from build123d import *

# Parameters (mm, degrees)
F1_DEPTH = 3.175
F2_R     = 5.08
F3_R     = 0.508


with BuildPart() as f1:
    # F0 (on Top) → F1 (new body)
    with BuildSketch(Plane.XY):
        with BuildLine():
            Line((-30.841844, 43.311745), (-30.841844, -61.686775))
            Line((-30.841844, -61.686775), (-18.141844, -61.686775))
            Line((-18.141844, -61.686775), (-5.441844, -23.358175))
            Line((-5.441844, -23.358175), (-5.441844, -10.658175))
            Line((-5.441844, -10.658175), (-18.141844, -10.658175))
            ThreePointArc((-18.141844, -10.658175), (-22.109324, -6.690695), (-18.141844, -2.723215))
            Line((-18.141844, -2.723215), (-5.441844, -2.723215))
            Line((-5.441844, -2.723215), (-5.441844, 0.451785))
            Line((-5.441844, 0.451785), (-18.141844, 0.451785))
            ThreePointArc((-18.141844, 0.451785), (-23.696824, 6.006765), (-18.141844, 11.561745))
            Line((-18.141844, 11.561745), (-5.441844, 11.561745))
            Line((-5.441844, 11.561745), (-5.441844, 17.911745))
            Line((-5.441844, 17.911745), (-18.141844, 17.911745))
            ThreePointArc((-18.141844, 17.911745), (-21.316844, 21.086745), (-18.141844, 24.261745))
            Line((-18.141844, 24.261745), (-5.441844, 24.261745))
            Line((-5.441844, 24.261745), (-5.441844, 27.436745))
            Line((-5.441844, 27.436745), (-18.141844, 27.436745))
            ThreePointArc((-18.141844, 27.436745), (-22.904344, 32.199245), (-18.141844, 36.961745))
            Line((-18.141844, 36.961745), (-5.441844, 36.961745))
            Line((-5.441844, 36.961745), (-5.441844, 43.311745))
            Line((-5.441844, 43.311745), (-30.841844, 43.311745))
        make_face()
    extrude(amount=F1_DEPTH)

    # F2
    f2_edges = [f1.edges().sort_by_distance(p)[0] for p in [
        (-18.141844, -61.686775, 1.5875),
        (-5.441844, -23.358175, 1.5875),
        (-30.841844, -61.686775, 1.5875),
        (-5.441844, 43.311745, 1.5875),
        (-30.841844, 43.311745, 1.5875),
    ]]
    fillet(f2_edges, radius=F2_R)

    # F3
    f3_edges = [f1.edges().sort_by_distance(p)[0] for p in [
        (-5.441844, -10.658175, 1.5875),
        (-5.441844, -2.723215, 1.5875),
        (-5.441844, 0.451785, 1.5875),
        (-5.441844, 11.561745, 1.5875),
        (-5.441844, 17.911745, 1.5875),
        (-5.441844, 24.261745, 1.5875),
        (-5.441844, 27.436745, 1.5875),
        (-5.441844, 36.961745, 1.5875),
    ]]
    fillet(f3_edges, radius=F3_R)


solid = f1.part
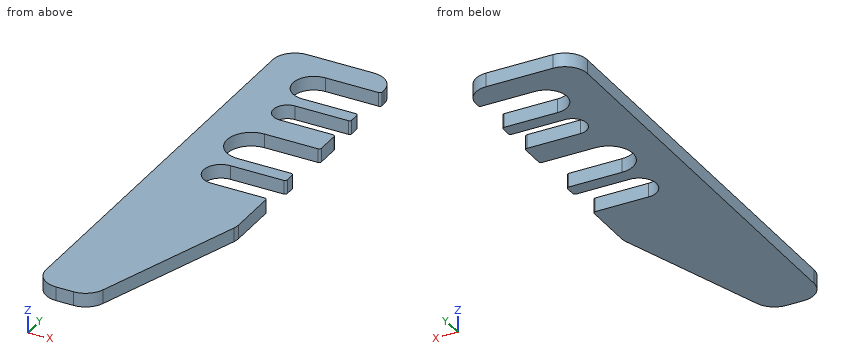
Read the model definition and answer for the solid it produces. Units are mm, in the model's axes. Coordinates: 2 decimals unless noted, no trailing zeros. Write each loop counter-clockwise with the first axis right and the second up, starting at its lowest first coordinate (ties: lowest second). Pieces come first, ordered by that corner, then holes. Notation, with made-up numbers: (-3, 45.25) -> (29, 45.25) arc R22 cw to (29, 82.25) -> close; hole circle Ø7 at (-28.5, -10). An arc over 180 degrees is marked (long way). Return JSON: item names as keys, results as strings.
(1) Consider line 1 along Y through (x, z) = (-19.75, 2.3); line 2 along Y through (x, z) = (-17.5, 2); line 3 along Y through (x, z) = (-21.75, 1.7). Determine where each line is inside the solid, lowest interval first. Write a range as from..to.
Answers below:
{"line 1": "-61.25..-10.32, -3.06..0.69, 11.32..18.35, 23.82..27.72, 36.68..43.31", "line 2": "-59.3..-10.66, -2.72..0.45, 11.56..17.91, 24.26..27.44, 36.96..43.31", "line 3": "-61.69..-8.34, -5.04..1.78, 10.23..29.09, 35.31..43.31"}
(2) Each of these flat-tipped pins is pushed along its axis until it touches: P1, Ø6, axis at x = -10.5, y = 11, coming from the +Z side (3 decimals); P2, Ø1, axis at x = -21, z = 2, coming from the -Y side. Where does it stop, or does it pass through?
Answers below:
{"P1": "z = 3.175", "P2": "y = -61.68"}
(3) The part is cut by section A-A on x = -20.25. Give the vertices of the cut face in (y, z) (3 decimals), then the cut area to 3 significant figures.
Answers below:
{"outline": "(-61.441, 0) -> (-10.052, 0) -> (-10.052, 3.175) -> (-61.441, 3.175) -> close; (-3.33, 0) -> (0.867, 0) -> (0.867, 3.175) -> (-3.33, 3.175) -> close; (11.146, 0) -> (18.713, 0) -> (18.713, 3.175) -> (11.146, 3.175) -> close; (23.461, 0) -> (27.929, 0) -> (27.929, 3.175) -> (23.461, 3.175) -> close; (36.47, 0) -> (43.312, 0) -> (43.312, 3.175) -> (36.47, 3.175) -> close", "area": "236 mm^2"}
(4) The part is cut by section C-C on x = -8.75. Give the vertices of the cut face in (y, z) (3 decimals), then the cut area to 3 significant figures.
Answers below:
{"outline": "(-33.342, 0) -> (-10.658, 0) -> (-10.658, 3.175) -> (-33.342, 3.175) -> close; (-2.723, 0) -> (0.452, 0) -> (0.452, 3.175) -> (-2.723, 3.175) -> close; (11.562, 0) -> (17.912, 0) -> (17.912, 3.175) -> (11.562, 3.175) -> close; (24.262, 0) -> (27.437, 0) -> (27.437, 3.175) -> (24.262, 3.175) -> close; (36.962, 0) -> (42.993, 0) -> (42.993, 3.175) -> (36.962, 3.175) -> close", "area": "131 mm^2"}
(5) The part is cut by section D-D on y = 28.5. Give the vertices of the cut face in (x, z) (3 decimals), then the cut area to 3 significant figures.
Answers below:
{"outline": "(-30.842, 0) -> (-21.141, 0) -> (-21.141, 3.175) -> (-30.842, 3.175) -> close", "area": "30.8 mm^2"}
